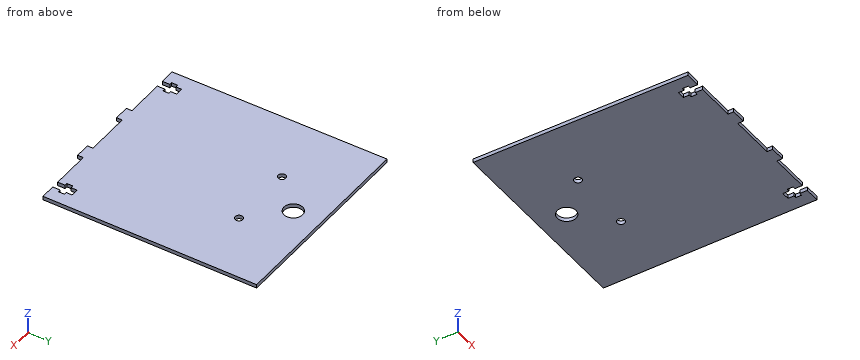
```python
from build123d import *

# Parameters (mm, degrees)
SKETCH_1_R      = 5.05
SKETCH_1_R_2    = 2.05
EXTRUDE_1_DEPTH = 2


with BuildPart() as part:
    # 草图1 → 凸台-拉伸1 (new body)
    with BuildSketch(Plane.XY):
        Polygon((-40.741188564, 3.13029316), (-40.741188564, 7.13029316), (-39.291188564, 7.13029316), (-39.291188564, 10.33029316), (-40.741188564, 10.33029316), (-40.741188564, 13.53029316), (-44.841188564, 13.53029316), (-44.841188564, 10.33029316), (-46.291188564, 10.33029316), (-46.291188564, 7.13029316), (-44.841188564, 7.13029316), (-44.841188564, 3.13029316), (-52.841188564, 3.13029316), (-53.870849739, 118.13029316), (43.582829756, 118.13029316), (53.258811436, 118.13029316), (53.258811436, 3.13029316), (45.258811436, 3.13029316), (45.258811436, 7.13029316), (46.708811436, 7.13029316), (46.708811436, 10.33029316), (45.258811436, 10.33029316), (45.258811436, 13.53029316), (41.158811436, 13.53029316), (41.158811436, 10.33029316), (39.708811436, 10.33029316), (39.708811436, 7.13029316), (41.158811436, 7.13029316), (41.158811436, 3.13029316), (20.208811436, 3.13029316), (20.208811436, 0.13029316), (12.208811436, 0.13029316), (12.208811436, 3.13029316), (-11.791188564, 3.13029316), (-11.791188564, 0.13029316), (-19.791188564, 0.13029316), (-19.791188564, 3.13029316), align=None)
        with Locations((0.208811436, 103.13029316)):
            Circle(SKETCH_1_R, mode=Mode.SUBTRACT)
        with Locations((17.886480965, 85.45262363)):
            Circle(SKETCH_1_R_2, mode=Mode.SUBTRACT)
        with Locations(Location((-17.468858094, 85.45262363, 0), (0, 0, 180))):
            Circle(SKETCH_1_R_2, mode=Mode.SUBTRACT)
    extrude(amount=EXTRUDE_1_DEPTH)


solid = part.part
```
Here's how the part is built. I have some questions about the finished solid (model axes, mm). Give positions to 0.01 mm unless a question says otherwise; leave off trailing zeros. Write each loop counter-clockwise with the first axis right and the second up, starting at its lowest first coordinate (ties: lowest second). Pieces come first, ordered by that corner, then holes. Notation, with made-up numbers: M -30,35 L -14,35 A19 cw -14,43 Z; hole C 80.25,-26.75 d2. An arc over 180 degrees is marked long. Put each result on its own line as item: value. Start each with the question number.
Item 1: If we section it at C-C, the plane z = 0.4: Count the separate pieces of the cut face and the enclosed holes in it, then the cut area to 3 significant figures.
Item 2: If we section it at B-B, the plane y = 100.5: Write out the boundary of the cut face in (x, z).
Item 3: If we section it at A-A, the plane x = -17.5: Write out the boundary of the cut face in (y, z), then the cut area to 3 significant figures.
Item 4: Will these pins go through, and if not, where does the flat tip stop? pin 1 (0.6 mm diameter, centred on y = 1, z = 1, fed in from -X); pin 2 (5.5 mm diameter, centred on x = -17.47, y = 85.45, fed in from -Z).
Item 5: I need wall thicknesses on L1, parallel to Y at x = -43, z = 1.9; L2, parallel to Y at x = -29, z = 0.25; L3, parallel to Y at x = 2.5, z = 0.75. Which ranges of each line are inside material? Lowest first, please. Write a range as from..to.
Item 6: If we section it at D-D, the plane x = 34: Write out the boundary of the cut face in (y, z), then the cut area to 3 significant figures.
Values:
1. separate pieces: 1
1. enclosed holes: 3
1. area: 12,100 mm²
2. outline: M -53.71,0 L -4.1,0 L -4.1,2 L -53.71,2 Z; M 4.52,0 L 53.26,0 L 53.26,2 L 4.52,2 Z
3. outline: M 0.13,0 L 83.4,0 L 83.4,2 L 0.13,2 Z; M 87.5,0 L 118.13,0 L 118.13,2 L 87.5,2 Z
3. area: 228 mm²
4. pin 1: x = -19.79
4. pin 2: z = 0
5. L1: 13.53..118.13
5. L2: 3.13..118.13
5. L3: 3.13..98.63, 107.63..118.13
6. outline: M 3.13,0 L 118.13,0 L 118.13,2 L 3.13,2 Z
6. area: 230 mm²
